Geometry check sheet. Reference: drawing and pictorial views, mm from the part's lowest x, y, z. Give positions to 0.01 mm unless a question says otherwise; leave off trailing zeros. Write each loop counter-clockwise with the first axis right and the second up, starting at its lowest first coordinate (ties: lowest second). Pieces come first, ordered by that corner, then holes. Notation, with made-up numbers: (72, 23.25) -> (88, 23.25) arc R37 ccw to (88, 61.25) -> close; hole circle Ø7 at (42, 28). An arc over 180 degrees is marked (long way). Answer as CSV lines item,"result".
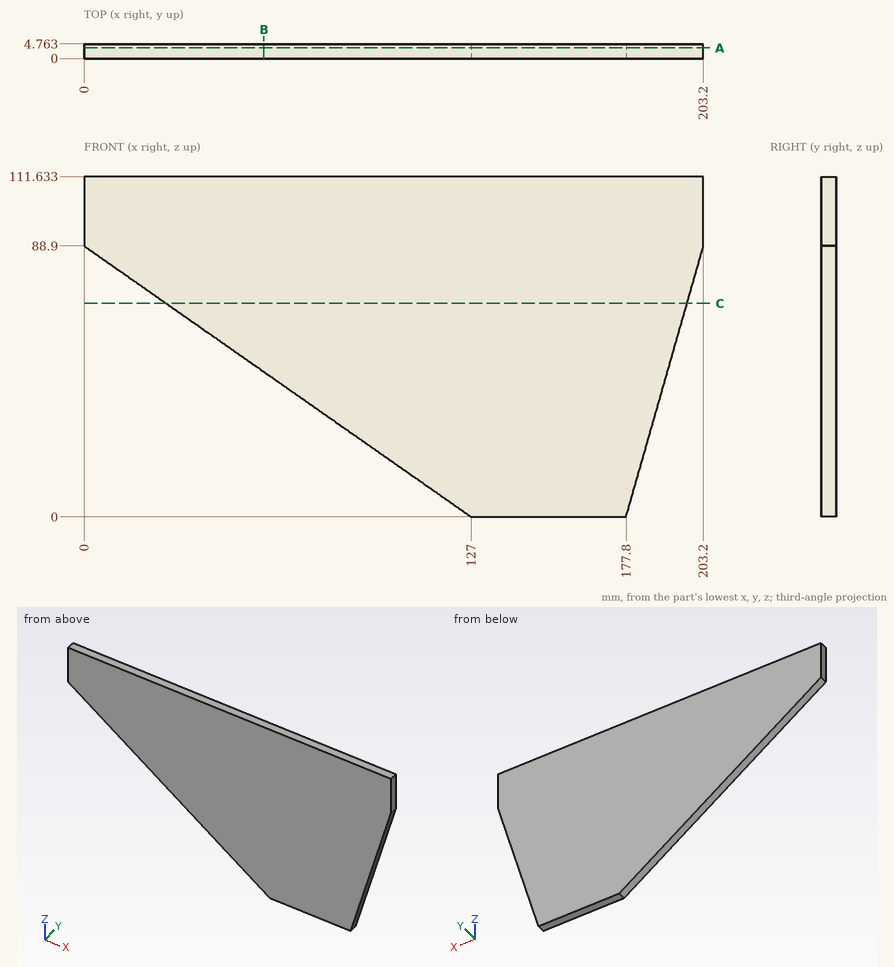
1) Depth check by flat-ended pin: pin 1 (12 mm diameter, centred on x = 92, z = 59.5, fed in from -Y); pin 2 (1.5 mm diameter, centred on x = 88.5, y = 2.5, fed in from -Z) (1 decimal). Enter the tip coordinate at first touch or a pass-through.
Reported:
pin 1,"y = 0"
pin 2,"z = 26.4"
2) Scan lines: line 1 along Z through (x, y) = (106, 4.05) (1 decimal); line 2 along X through (y, z) = (1.05, 30.5) (1 decimal); line 3 along X through (y, z) = (3.45, 84). Record each from-to range of solid material in increasing order.
Reported:
line 1,"14.7 to 111.6"
line 2,"83.4 to 186.5"
line 3,"7 to 201.8"
3) Section check C-C (z = 70). Record the boundary of the cut face in (x, y).
Reported:
outline,"(27, 0) -> (197.8, 0) -> (197.8, 4.76) -> (27, 4.76) -> close"
4) Section check B-B (x = 59). Record the boundary of the cut face in (y, z), and give its area (3 significant figures).
Reported:
outline,"(0, 47.6) -> (4.76, 47.6) -> (4.76, 111.63) -> (0, 111.63) -> close"
area,"305 mm²"
5) Section check A-A (y = 3.5). Record the boundary of the cut face in (x, z), and give its area (3 significant figures).
Reported:
outline,"(0, 88.9) -> (127, 0) -> (177.8, 0) -> (203.2, 88.9) -> (203.2, 111.63) -> (0, 111.63) -> close"
area,"15,900 mm²"
